Source: CAD feature listing. Evaluate the final solid. Frame: model axes, mm. A direction names the side the tool comes from. Give positions to 0.01 mm unless a question says otherwise; leave off trailing zeros. Order: outer loops, then holes, each group sorted by start corner. A loop starts at its lowest first (then second) coordinate and runs counter-clockwise, first axis right, second up. Notation, with made-up numbers: (70.5, 85) - (81.5, 85) arc R18 ccw to (81.5, 118) - close; hole circle Ø10 at (-25.5, 7). An arc over 180 degrees is marked (long way). Answer as CSV lines item,"result".
```python
from build123d import *

# Parameters (mm, degrees)
SKETCH1_R           = 36
SKETCH1_R_2         = 3.5
SKETCH1_R_3         = 1.65
BOSS_EXTRUDE1_DEPTH = 4
SKETCH2_R           = 14.5
BOSS_EXTRUDE2_DEPTH = 6.5
SKETCH3_R           = 36
SKETCH3_R_2         = 33
BOSS_EXTRUDE3_DEPTH = 8
CHAMFER1_SIZE       = 1.6


with BuildPart() as part:
    # Sketch1 → Boss-Extrude1 (new body)
    with BuildSketch(Plane(origin=(0, 0, 0), x_dir=(1, 0, 0), z_dir=(0, 1, 0))):
        Circle(SKETCH1_R)
        with Locations((25, 0)):
            Circle(SKETCH1_R_2, mode=Mode.SUBTRACT)
        with Locations((0, -25)):
            Circle(SKETCH1_R_2, mode=Mode.SUBTRACT)
        with Locations((-10, 20)):
            Circle(SKETCH1_R_3, mode=Mode.SUBTRACT)
        with Locations((10, 20)):
            Circle(SKETCH1_R_3, mode=Mode.SUBTRACT)
        with Locations((10, -20)):
            Circle(SKETCH1_R_3, mode=Mode.SUBTRACT)
        with Locations((-10, -20)):
            Circle(SKETCH1_R_3, mode=Mode.SUBTRACT)
        with Locations((0, 25)):
            Circle(SKETCH1_R_2, mode=Mode.SUBTRACT)
        with Locations((-25, 0)):
            Circle(SKETCH1_R_2, mode=Mode.SUBTRACT)
    extrude(amount=BOSS_EXTRUDE1_DEPTH)

    # Sketch2 → Boss-Extrude2 (add)
    with BuildSketch(Plane(origin=(0, 4, 0), x_dir=(1, 0, 0), z_dir=(0, 1, 0))):
        Circle(SKETCH2_R)
    extrude(amount=BOSS_EXTRUDE2_DEPTH)

    # Sketch3 → Boss-Extrude3 (add)
    with BuildSketch(Plane(origin=(0, 4, 0), x_dir=(1, 0, 0), z_dir=(0, 1, 0))):
        Circle(SKETCH3_R)
        Circle(SKETCH3_R_2, mode=Mode.SUBTRACT)
    extrude(amount=BOSS_EXTRUDE3_DEPTH)

    # Chamfer1
    chamfer1_edges = [part.edges().sort_by_distance(p)[0] for p in [
        (8.35, 4, -20),
        (8.35, 4, 20),
        (-11.65, 4, 20),
        (-11.65, 4, -20),
    ]]
    chamfer(chamfer1_edges, length=CHAMFER1_SIZE)


solid = part.part
```
(1) Mould query, pull axis X, two halves, no side actions, for faces 1 (the cylindrical face through (10.89, 1.18, -21.39)), 2 (the cylindrical face through (-4.686, 5.916, -35.694)), 3 (the cylindrical face through (-9.11, 1.18, 18.61)), 4 (the flat face through (15.8, 12, 29.2)). Classes: released by +X, released by -X, zero draft, split by the parting line, or undercut.
Completed:
face 1,"undercut"
face 2,"split by the parting line"
face 3,"undercut"
face 4,"zero draft"
(2) Cut plane A-A (z = 0). Return loops of the section in (x, y).
Completed:
outline,"(-36, 0) - (-28.5, 0) - (-28.5, 4) - (-33, 4) - (-33, 12) - (-36, 12) - close; (-21.5, 0) - (21.5, 0) - (21.5, 4) - (14.5, 4) - (14.5, 10.5) - (-14.5, 10.5) - (-14.5, 4) - (-21.5, 4) - close; (28.5, 0) - (36, 0) - (36, 12) - (33, 12) - (33, 4) - (28.5, 4) - close"
(3) Cut plane B-B (x = 25). Return loops of the section in (y, z), then the cut area to 3 significant figures.
Completed:
outline,"(0, -25.9) - (12, -25.9) - (12, -21.54) - (4, -21.54) - (4, -3.5) - (0, -3.5) - close; (0, 3.5) - (4, 3.5) - (4, 21.54) - (12, 21.54) - (12, 25.9) - (0, 25.9) - close"
area,"249 mm²"
(4) Cut plane C-C (y = 6.75). Return loops of the section in (x, z).
Completed:
outline,"circle Ø72 at (0, 0); circle Ø29 at (0, 0); hole circle Ø66 at (0, 0)"
(5) Access query for faces 5 (the flat face through (-1, 0, -1)), 6 (the flat face through (0, 10.5, 0)). Directions: +Z, -Z, +X, -X, +Y, -Y. A direction counts if a zero-diameter tool reaches every point of the face in a straight line with its end or side. Return the directions, or none.
Completed:
face 5,"+Z, -Z, +X, -X, -Y"
face 6,"+Y"
(6) Contact query for flat-ended pins moving along their axis: pin 1 (4 mm diameter, centred on x = -5.5, z = 11, fed in from +Y); pin 2 (1.5 mm diameter, centred on y = 7.5, z = -10.5, fed in from +X); pin 3 (3 mm diameter, centred on x = -10, z = 20, fed in from +Y); pin 4 (5 mm diameter, centred on x = 11.5, y = 3.5, fed in from -Z). Output: stop coordinate, or through.
Completed:
pin 1,"y = 10.5"
pin 2,"x = 34.65"
pin 3,"through"
pin 4,"z = -34.86"
(7) Ray query, line 1 (Z direction, x = 0, y = 6.5); line 2 (X direction, y = 8, z = -10.5). Return the intervals inside material, ascending. Write a range as from..to.
Completed:
line 1,"-36..-33, -14.5..14.5, 33..36"
line 2,"-34.43..-31.28, -10..10, 31.28..34.43"
(8) Cut plane D-D (z = -25). Return loops of the section in (x, y).
Completed:
outline,"(-25.9, 0) - (-3.5, 0) - (-3.5, 4) - (-21.54, 4) - (-21.54, 12) - (-25.9, 12) - close; (3.5, 0) - (25.9, 0) - (25.9, 12) - (21.54, 12) - (21.54, 4) - (3.5, 4) - close"
